Can you work these out from the model? Positions are in its coordinate system, mm. Face numbers are marked on the shaded views. A direction names the side the tool comes from. Coordinates: 2 decimals unless noted, no trailing zeros. Order: outer loops, then holes, each group sorted by start corner. A loop starts at its lowest first (then second) coordinate and runs counter-clockwise, first axis right, second up.
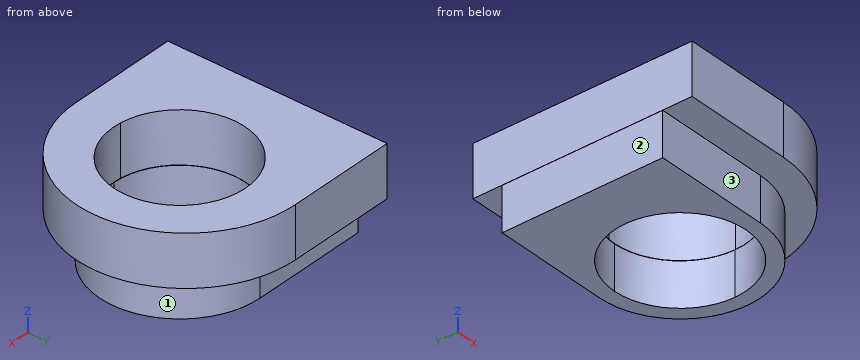
```python
from build123d import *

# Parameters (mm, degrees)
F1_DEPTH = 3.5
F3_DEPTH = 3


with BuildPart() as f1:
    # F0 (on Top) → F1 (new body)
    with BuildSketch(Plane.XY):
        with BuildLine():
            Line((-41.077644, 41.93693), (-48.577644, 41.93693))
            Line((-48.577644, 41.93693), (-48.577644, 26.93693))
            Line((-48.577644, 26.93693), (-41.077644, 26.93693))
            Line((-41.077644, 26.93693), (-41.077644, 29.964794))
            ThreePointArc((-41.077644, 29.964794), (-45.077644, 34.43693), (-41.077644, 38.909066))
            Line((-41.077644, 38.909066), (-41.077644, 41.93693))
        make_face()
        with BuildLine():
            ThreePointArc((-41.077644, 26.93693), (-33.577644, 34.43693), (-41.077644, 41.93693))
            Line((-41.077644, 41.93693), (-41.077644, 38.909066))
            ThreePointArc((-41.077644, 38.909066), (-37.577644, 37.791032), (-36.077644, 34.43693))
            ThreePointArc((-36.077644, 34.43693), (-37.577644, 31.082828), (-41.077644, 29.964794))
            Line((-41.077644, 29.964794), (-41.077644, 26.93693))
        make_face()
    extrude(amount=F1_DEPTH)

    # F2 (on Top) → F3 (join)
    with BuildSketch(Plane.XY):
        with BuildLine():
            Line((-40.561818, 39.95863), (-48.561818, 39.95863))
            Line((-48.561818, 39.95863), (-48.561818, 28.95863))
            Line((-48.561818, 28.95863), (-40.561818, 28.95863))
            Line((-40.561818, 28.95863), (-40.561818, 29.95863))
            ThreePointArc((-40.561818, 29.95863), (-45.061818, 34.45863), (-40.561818, 38.95863))
            Line((-40.561818, 38.95863), (-40.561818, 39.95863))
        make_face()
        with BuildLine():
            ThreePointArc((-40.561818, 28.95863), (-35.061818, 34.45863), (-40.561818, 39.95863))
            Line((-40.561818, 39.95863), (-40.561818, 38.95863))
            ThreePointArc((-40.561818, 38.95863), (-37.379837, 37.64061), (-36.061818, 34.45863))
            ThreePointArc((-36.061818, 34.45863), (-37.379837, 31.276649), (-40.561818, 29.95863))
            Line((-40.561818, 29.95863), (-40.561818, 28.95863))
        make_face()
    extrude(amount=-F3_DEPTH)


solid = f1.part
```
1. Imagine slicing it at A-A on z = -1.75. Please give me the cut outline in (x, y).
Completed:
outline: (-48.56, 28.96) - (-40.56, 28.96) arc R5.5 ccw to (-40.56, 39.96) - (-48.56, 39.96) - close; hole (-40.56, 29.96) arc R4.5 ccw to (-36.06, 34.46) arc R4.5 ccw (long way) to start
2. Imagine slicing it at D-D on x = -46. Please give me the cut outline in (y, z).
Completed:
outline: (26.94, 0) - (28.96, 0) - (28.96, -3) - (39.96, -3) - (39.96, 0) - (41.94, 0) - (41.94, 3.5) - (26.94, 3.5) - close
3. I'm going to push flat-ended pins straight in: pin 1 (3.5 mm diameter, centred on x = -39, y = 33.5, fed in from +Z); pin 2 (0.9 mm diameter, centred on y = 36, z = -1, fed in from -X); pin 3 (3 mm diameter, centred on x = -37.5, z = 2.5, fed in from +Y); pin 4 (1.5 mm diameter, centred on x = -41.5, z = -1, fed in from -Y). Where does each tip first touch, or does it pass through?
Completed:
pin 1: passes through
pin 2: stops at x = -48.56
pin 3: stops at y = 41.64
pin 4: stops at y = 28.96
4. Please list where these lines run through material, in increasing order: probe 1 along Y at (x, z) = (-48, -2.5); probe 2 along X at (y, z) = (35.75, 1.75); probe 3 along Z at (x, y) = (-36.5, 39.25).
Completed:
probe 1: y = 28.96 to 39.96
probe 2: x = -48.58 to -44.88, -36.27 to -33.69
probe 3: z = 0 to 3.5
5. On a 3-axis mill with a long thin cutter (end or side, diameter ignored), from which of +Z, -Z, +X, -X, +Y, -Y can I reach the whole of each face in a straight line? I mean the marked faces 1, 2 and 3. Say none if no direction works.
Completed:
face 1: -Z, +X
face 2: -Z, -X, +Y, -Y
face 3: -Z, +X, -X, -Y
